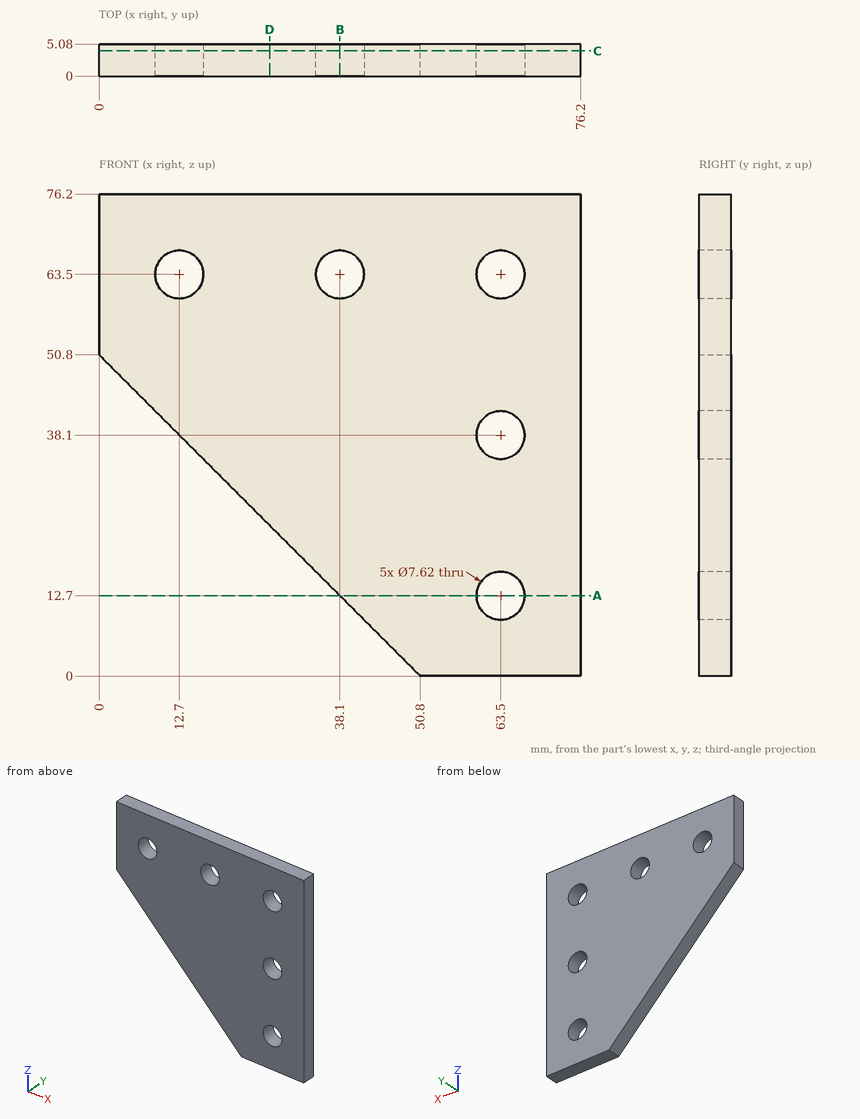
Source: three-view drawing plus pictorial views. Frame: mm from the lowest corner of the part. Round coordinates to 2 decimals unless told otherwise and drop trailing zeros. Loops run counter-clockwise (first coordinate to the right, second up) from the corner with the lowest first, then second, coordinate; pieces in that order, holes last. Notation, with made-up numbers: (53.25, 62) - (102.25, 62) arc R19 cw to (102.25, 79) - close; hole circle Ø4 at (56, 16.5). An arc over 180 degrees is marked (long way). Write item = value, one per line. Start each with the question number.
Item 1: Section query D-D on x = 27. Output: boundary loops of the cut face in (y, z).
Item 2: Section query C-C on y = 4. Output: boundary loops of the cut face in (x, z).
Item 3: Section query B-B on x = 38.1. Output: boundary loops of the cut face in (y, z), plus the area to 3 significant figures.
Item 4: Section query A-A on z = 12.7. Output: boundary loops of the cut face in (x, y).
Item 5: Material intervals for line 1 (Z direction, x = 63.5, y = 3.45); line 2 (Z direction, x = 67, y = 1.5); line 3 (X direction, y = 4.85, z = 61), sorted ascending.
Item 6: First-contact query: pin 1 Ø1 at (y, z) = (4, 9) entering from -X; pin 2 Ø6 at (x, z) = (38.1, 63.5) entering from +Y; pin 3 Ø1 at (x, y) = (34.5, 4) entering from -Z. Flat tips, straight axial feed; report the tip coordinate or a pass-through.
Results list:
q1.outline = (0, 23.8) - (5.08, 23.8) - (5.08, 76.2) - (0, 76.2) - close
q2.outline = (0, 50.8) - (50.8, 0) - (76.2, 0) - (76.2, 76.2) - (0, 76.2) - close; hole circle Ø7.62 at (12.7, 63.5); hole circle Ø7.62 at (38.1, 63.5); hole circle Ø7.62 at (63.5, 12.7); hole circle Ø7.62 at (63.5, 38.1); hole circle Ø7.62 at (63.5, 63.5)
q3.outline = (0, 12.7) - (5.08, 12.7) - (5.08, 59.69) - (0, 59.69) - close; (0, 67.31) - (5.08, 67.31) - (5.08, 76.2) - (0, 76.2) - close
q3.area = 284 mm²
q4.outline = (38.1, 0) - (59.69, 0) - (59.69, 5.08) - (38.1, 5.08) - close; (67.31, 0) - (76.2, 0) - (76.2, 5.08) - (67.31, 5.08) - close
q5.line_1 = 0 to 8.89, 16.51 to 34.29, 41.91 to 59.69, 67.31 to 76.2
q5.line_2 = 0 to 11.19, 14.21 to 36.59, 39.61 to 61.99, 65.01 to 76.2
q5.line_3 = 0 to 9.82, 15.58 to 35.22, 40.98 to 60.62, 66.38 to 76.2
q6.pin_1 = 41.3
q6.pin_2 = through
q6.pin_3 = 15.8
